Could you check a few things on this model? Use its own coordinates, in mm. Face numbers are marked on the shaded views. A direction names the side the tool comes from. Coordinates: 2 decimals unless noted, no trailing zeros. Loops run counter-clockwise (first coordinate to the right, second up) from the corner with the lowest first, then second, coordinate; pieces in that order, holes last. Notation, with made-up numbers: (-1.75, 1) - (3.25, 1) arc R30 cw to (3.25, 27) - close; hole circle Ø9 at (64.25, 78.5). An arc over 180 degrees is marked (long way). One line per item, written item: value. Start each with the question number.
(1) If we section it at C-C on z = 7.5: Write out the boundary of the cut face in (x, y).
(2) If we section it at D-D on y = 12: Write out the boundary of the cut face in (x, z).
(3) On a 3-axis mill with a long thin cutter (end or side, diameter ignored), from which of +Z, -Z, +X, -X, +Y, -Y can I reach the whole of each face in a straight line? I mean the marked faces 1 and 2. Say none if no direction works.
(4) If we section it at B-B on x = 30: Write out the boundary of the cut face in (y, z).
(5) If we section it at A-A on y = 0: Write out the boundary of the cut face in (x, z).
(6) If I drill on line 1 along X through (y, z) = (0, 2.05); line 2 along Z through (x, y) = (5.5, 0); line 3 along Y through (x, z) = (2, 9.5), over which ranges is the centre line in solid material (lowest first)? Write a range as from..to.
(7) I'm going to push flat-ended pins straight in: P1, Ø7, axis at y = 0, z = 9, coming from the -X side; P2, Ø8, axis at y = 19.5, z = 4, coming from the +X side; P3, Ø1, axis at x = 15, y = -5, coming from the +Z side; P4, Ø2.5, axis at x = 15, y = 0, coming from the +Z side. Where does each tip first touch, or does it pass through?
(8) If we mould it in two halves opening along X, with no side actions, what happens to the marked faces 3, 4 and 5? For each: pulls with the +X half, pulls with the -X half, needs draft (parallel to the pull), parting line crosses it, or undercut.
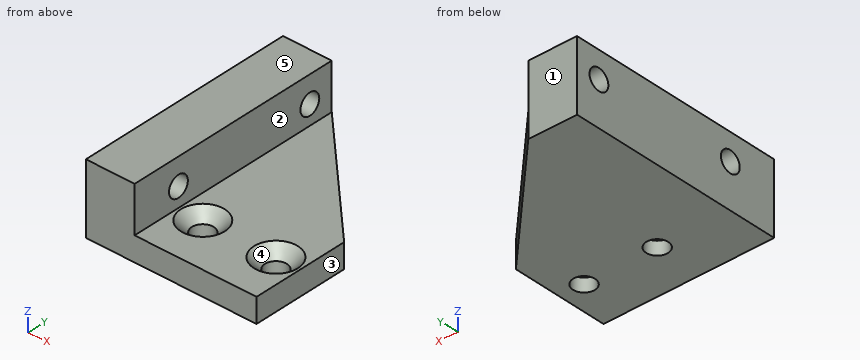
```python
from build123d import *

# Parameters (mm, degrees)
SKETCH033_R         = 2.25
PAD019_DEPTH        = 5
SKETCH035_W         = 45
SKETCH035_H         = 14.5
SKETCH035_R         = 2.15
PAD020_DEPTH        = 10
HOLE007_D           = 4.5
HOLE007_CSINK_D     = 9
HOLE007_CSINK_ANGLE = 90


with BuildPart() as part:
    # Sketch033 → Pad019 (new body)
    with BuildSketch(Plane.XY):
        Polygon((35, 10), (35, -10), (0, -10), (0, 35), (10, 35), align=None)
        with Locations((15, 0)):
            Circle(SKETCH033_R, mode=Mode.SUBTRACT)
        with Locations((30, 0)):
            Circle(SKETCH033_R, mode=Mode.SUBTRACT)
    extrude(amount=PAD019_DEPTH)

    # Sketch035 → Pad020 (join)
    with BuildSketch(Plane.YZ):
        with Locations((12.5, 7.25)):
            Rectangle(SKETCH035_W, SKETCH035_H)
        with Locations((0, 9)):
            Circle(SKETCH035_R, mode=Mode.SUBTRACT)
        with Locations((30, 9)):
            Circle(SKETCH035_R, mode=Mode.SUBTRACT)
    extrude(amount=PAD020_DEPTH)

    # Hole007 (through all)
    with Locations(Plane.XY.offset(5)):
        with Locations((15, 0), (30, 0)):
            CounterSinkHole(HOLE007_D / 2, HOLE007_CSINK_D / 2, counter_sink_angle=HOLE007_CSINK_ANGLE)


solid = part.part
```
Values:
1. outline: (0, -10) - (10, -10) - (10, -1.54) - (0, -1.54) - close; (0, 1.54) - (10, 1.54) - (10, 28.46) - (0, 28.46) - close; (0, 31.54) - (10, 31.54) - (10, 35) - (0, 35) - close
2. outline: (0, 0) - (33, 0) - (33, 5) - (10, 5) - (10, 14.5) - (0, 14.5) - close
3. face 1: +Z, -Z, +X, -X, +Y
3. face 2: +Z, +X, +Y, -Y
4. outline: (-10, 0) - (-2.25, 0) - (-2.25, 2.75) - (-4.5, 5) - (-10, 5) - close; (2.25, 0) - (15, 0) - (15, 5) - (4.5, 5) - (2.25, 2.75) - close
5. outline: (0, 0) - (12.75, 0) - (12.75, 2.75) - (10.5, 5) - (10, 5) - (10, 6.85) - (0, 6.85) - close; (0, 11.15) - (10, 11.15) - (10, 14.5) - (0, 14.5) - close; (17.25, 0) - (27.75, 0) - (27.75, 2.75) - (25.5, 5) - (19.5, 5) - (17.25, 2.75) - close; (32.25, 0) - (35, 0) - (35, 5) - (34.5, 5) - (32.25, 2.75) - close
6. line 1: x = 0..12.75, 17.25..27.75, 32.25..35
6. line 2: z = 0..6.85, 11.15..14.5
6. line 3: y = -10..-2.09, 2.09..27.91, 32.09..35
7. P1: stops at x = 0
7. P2: stops at x = 29.5
7. P3: stops at z = 5
7. P4: passes through
8. face 3: pulls with the +X half
8. face 4: undercut
8. face 5: needs draft
